Check sheet for the modelled part. Datum: model origin and axes. Units: mm. A direction names the side the tool comes from. Give positions to 0.01 mm unless a question says otherwise; leave off trailing zeros. Write each question's results on one line, items separated by ' | '. Start each with the question number.
1. Gauge pin test, flat ends, axial feed: pin 1 Ø3 at (y, z) = (-12.5, 43) entering from -X; pin 2 Ø2.5 at (x, z) = (11, 47) entering from -Y; pin 3 Ø2 at (y, z) = (-30.5, 34.5) entering from +X; pin 4 Ø7 at (x, y) = (19.28, 22.98) entering from -Z. Record the tip position at first contact, or that the pin passes through.
2. Tool access check on faces 3 (the face through (-9.114, -5.214, 47.098)), 4 (the face through (-10, -6, 54)). Record the directions out of +Z, -Z, +X, -X, +Y, -Y that give a thin tool (end or side, any length) a straight path to the whole face; none if there is none.
3. Material ranges on L1, parallel to Y at x = 0, z = 5; L2, parallel to Y at x = 0, z = 0.95; L3, parallel to X at y = -27, z = 37.5, recorded low to high. Write a range as from..to.
4. Cross-section at A-A on z = 41.5. Count the separate pieces of the cut face and the enclosed holes in it, and give its area (3 significant figures).
5. Mould release check, pull along X, two halves, no side actions. Record for faces 1 (the face through (-22.39, 7.46, 27.24)), 2 (the face through (-34.2, -26.224, 35.514)): +X half, -X half, draft (parallel to the pull), parting line (faces both ways), or undercut.
from build123d import *

# Parameters (mm, degrees)
SKETCH_1_R                           = 37.5
EXTRUDE_1_DEPTH                      = 2
SKETCH_2_R                           = 45
EXTRUDE_2_DEPTH                      = 24
SKETCH_3_R                           = 43
EXTRUDE_3_DEPTH                      = 10
SKETCH_4_R                           = 43
EXTRUDE_4_DEPTH                      = 10
SKETCH_7_R                           = 7.5
CUT_EXTRUDE_1_DEPTH                  = 36
SKETCH_8_R                           = 3
CUT_EXTRUDE_2_DEPTH                  = 87.104587567
CHAMFER_1_SIZE                       = 2
PATTERN_CIRCULAR_1_COUNT             = 9
CHAMFER_1_OF_PATTERN_CIRCULAR_1_SIZE = 2
SKETCH_9_R                           = 12.5
CUT_EXTRUDE_3_DEPTH                  = 14
CUT_EXTRUDE_4_DEPTH                  = 84.462566459
PATTERN_CIRCULAR_2_COUNT             = 3
SKETCH_11_R                          = 10.5
CUT_EXTRUDE_5_DEPTH                  = 94.134311615
SKETCH_12_R                          = 22.5
CUT_EXTRUDE_6_DEPTH                  = 2
SKETCH_13_R                          = 16
CUT_EXTRUDE_7_DEPTH                  = 3.5
SKETCH_14_R                          = 17.85
CUT_EXTRUDE_8_DEPTH                  = 1.5
SKETCH_15_R                          = 16
CUT_EXTRUDE_9_DEPTH                  = 40


# Read off the part's stored shape, not the designer's step: 边界1
with BuildPart() as part:
    # 草图1 → 凸台-拉伸1 (new body)
    with BuildSketch(Plane.XY):
        Circle(SKETCH_1_R)
    extrude(amount=EXTRUDE_1_DEPTH)

    # 草图2 → 凸台-拉伸2 (add)
    with BuildSketch(Plane.XY.offset(2)):
        Circle(SKETCH_2_R)
    extrude(amount=EXTRUDE_2_DEPTH)

    # 草图3 → 凸台-拉伸3 (add)
    with BuildSketch(Plane.XY.offset(26)):
        Circle(SKETCH_3_R)
    extrude(amount=EXTRUDE_3_DEPTH)

    # 边界1 outline → 边界1 (revolve)
    with BuildSketch(Plane.XZ):
        Polygon((45, 26), (43, 36), (43, 26), align=None)
    revolve(axis=Axis((0, 0, 0), (0, 0, 1)))

    # 草图4 → 凸台-拉伸4 (add)
    with BuildSketch(Plane.XY.offset(36)):
        Circle(SKETCH_4_R)
    extrude(amount=EXTRUDE_4_DEPTH)

    # 草图6 → 旋转1 (revolve)
    with BuildSketch(Plane(origin=(0, 0, 0), x_dir=(0, 0, -1), z_dir=(1, 0, 0)), mode=Mode.PRIVATE) as revolve_1_sk:
        with BuildLine():
            Line((-46, 0), (-46, 17.5))
            Line((-46, 17.5), (-58.202041029, 17.5))
            ThreePointArc((-58.202041029, 17.5), (-63.325516412, 16.733200531), (-68, 14.5))
            Line((-68, 14.5), (-68, 0))
            Line((-68, 0), (-46, 0))
        make_face()
    revolve(revolve_1_sk.sketch.rotate(Axis((0, 0, 46), (0, 0, 1)), 90), axis=Axis((0, 0, 46), (0, 0, 1)))

    # 草图7 → 切除-拉伸1 (cut)
    with BuildSketch(Plane.XY.offset(46)):
        with Locations((0, 30)):
            Circle(SKETCH_7_R)
    cut_extrude_1 = extrude(amount=-CUT_EXTRUDE_1_DEPTH, mode=Mode.SUBTRACT)

    # 草图8 → 切除-拉伸2 (cut, through all)
    with BuildSketch(Plane.XY.offset(10)):
        with Locations((0, 30)):
            Circle(SKETCH_8_R)
    cut_extrude_2 = extrude(amount=-CUT_EXTRUDE_2_DEPTH, mode=Mode.SUBTRACT)

    # 倒角1
    chamfer_1_edges = [part.edges().sort_by_distance(p)[0] for p in [
        (-7.5, 30, 46),
        (-3, 30, 10),
    ]]
    chamfer(chamfer_1_edges, length=CHAMFER_1_SIZE)

    # 阵列(圆周)1: 切除-拉伸1, 切除-拉伸2 ×9 about axis
    pattern_circular_1_axis = Axis((0, 0, 0), (0, 0, 1))
    add([cut_extrude_1.rotate(pattern_circular_1_axis, i * 360 / PATTERN_CIRCULAR_1_COUNT) for i in range(1, PATTERN_CIRCULAR_1_COUNT)], mode=Mode.SUBTRACT)
    add([cut_extrude_2.rotate(pattern_circular_1_axis, i * 360 / PATTERN_CIRCULAR_1_COUNT) for i in range(1, PATTERN_CIRCULAR_1_COUNT)], mode=Mode.SUBTRACT)

    # 倒角1 of 阵列(圆周)1
    chamfer_1_of_pattern_circular_1_edges = [part.edges().sort_by_distance(p)[0] for p in [
        (-25.028961614, 18.160426221, 46),
        (-21.58176162, 21.052970465, 10),
        (-30.846593923, -2.176612818, 46),
        (-30.065177123, 2.255022071, 10),
        (-22.230762114, -21.495190528, 46),
        (-24.480762114, -17.598076211, 10),
        (-3.212909644, -30.755929699, 46),
        (-7.441526437, -29.216839054, 10),
        (17.308298956, -25.625627549, 46),
        (13.079682162, -27.164718194, 10),
        (29.730762114, -8.504809472, 46),
        (27.480762114, -12.401923789, 10),
        (28.241871258, 12.595503478, 46),
        (29.023288057, 8.163868589, 10),
        (13.538294967, 27.802240366, 46),
        (16.985494961, 24.909696123, 10),
    ]]
    chamfer(chamfer_1_of_pattern_circular_1_edges, length=CHAMFER_1_OF_PATTERN_CIRCULAR_1_SIZE)

    # 草图9 → 切除-拉伸3 (cut)
    with BuildSketch(Plane.XY.offset(68)):
        Circle(SKETCH_9_R)
    extrude(amount=-CUT_EXTRUDE_3_DEPTH, mode=Mode.SUBTRACT)

    # 草图10 → 切除-拉伸4 (cut, through all)
    with BuildSketch(Plane.XY.offset(54)):
        with BuildLine():
            Line((-12.247448714, -2.5), (12.247448714, -2.5))
            ThreePointArc((12.247448714, -2.5), (12.5, 0), (12.247448714, 2.5))
            Line((12.247448714, 2.5), (-12.247448714, 2.5))
            ThreePointArc((-12.247448714, 2.5), (-12.5, 0), (-12.247448714, -2.5))
        make_face()
    cut_extrude_4 = extrude(amount=-CUT_EXTRUDE_4_DEPTH, mode=Mode.SUBTRACT)

    # 阵列(圆周)2: 切除-拉伸4 ×3 about axis
    pattern_circular_2_axis = Axis((0, 0, 0), (0, 0, 1))
    for i in range(1, PATTERN_CIRCULAR_2_COUNT):
        add(cut_extrude_4.rotate(pattern_circular_2_axis, i * 360 / PATTERN_CIRCULAR_2_COUNT), mode=Mode.SUBTRACT)

    # 草图11 → 切除-拉伸5 (cut, through all)
    with BuildSketch(Plane.XY.offset(68)):
        Circle(SKETCH_11_R)
    extrude(amount=-CUT_EXTRUDE_5_DEPTH, mode=Mode.SUBTRACT)

    # 草图12 → 切除-拉伸6 (cut)
    with BuildSketch(Plane(origin=(0, 0, 0), x_dir=(-1, 0, 0), z_dir=(0, 0, -1))):
        Circle(SKETCH_12_R)
    extrude(amount=-CUT_EXTRUDE_6_DEPTH, mode=Mode.SUBTRACT)

    # 草图13 → 切除-拉伸7 (cut)
    with BuildSketch(Plane(origin=(0, 0, 2), x_dir=(-1, 0, 0), z_dir=(0, 0, -1))):
        Circle(SKETCH_13_R)
    extrude(amount=-CUT_EXTRUDE_7_DEPTH, mode=Mode.SUBTRACT)

    # 草图14 → 切除-拉伸8 (cut)
    with BuildSketch(Plane(origin=(0, 0, 5.5), x_dir=(-1, 0, 0), z_dir=(0, 0, -1))):
        Circle(SKETCH_14_R)
    extrude(amount=-CUT_EXTRUDE_8_DEPTH, mode=Mode.SUBTRACT)

    # 草图15 → 切除-拉伸9 (cut)
    with BuildSketch(Plane(origin=(0, 0, 0), x_dir=(-1, 0, 0), z_dir=(0, 0, -1))):
        Circle(SKETCH_15_R)
    extrude(amount=-CUT_EXTRUDE_9_DEPTH, mode=Mode.SUBTRACT)


solid = part.part
Geometry says:
1) pin 1: x = -41.57 | pin 2: y = -41.76 | pin 3: x = 31.74 | pin 4: z = 0
2) face 3: +Z, -Z | face 4: +Z
3) L1: -45..-16, 16..27, 33..45 | L2: -37.5..-22.5, 22.5..27, 33..37.5 | L3: -33.47..-17.67, -2.86..2.86, 17.67..33.47
4) separate pieces: 1 | enclosed holes: 10 | area: 3,810 mm^2
5) face 1: undercut | face 2: parting line
